Check sheet for the drawn part. Datum: minimum x, y, z corner. Units: mm. A direction names the side the tool comes from. Give positions to 0.01 mm unless a question says otherwise; leave off trailing zeros. Order: outer loops, then holes, each group sorted by start corner. A loop starts at its lowest first (then second) coordinate and runs counter-clockwise, first axis right, second up.
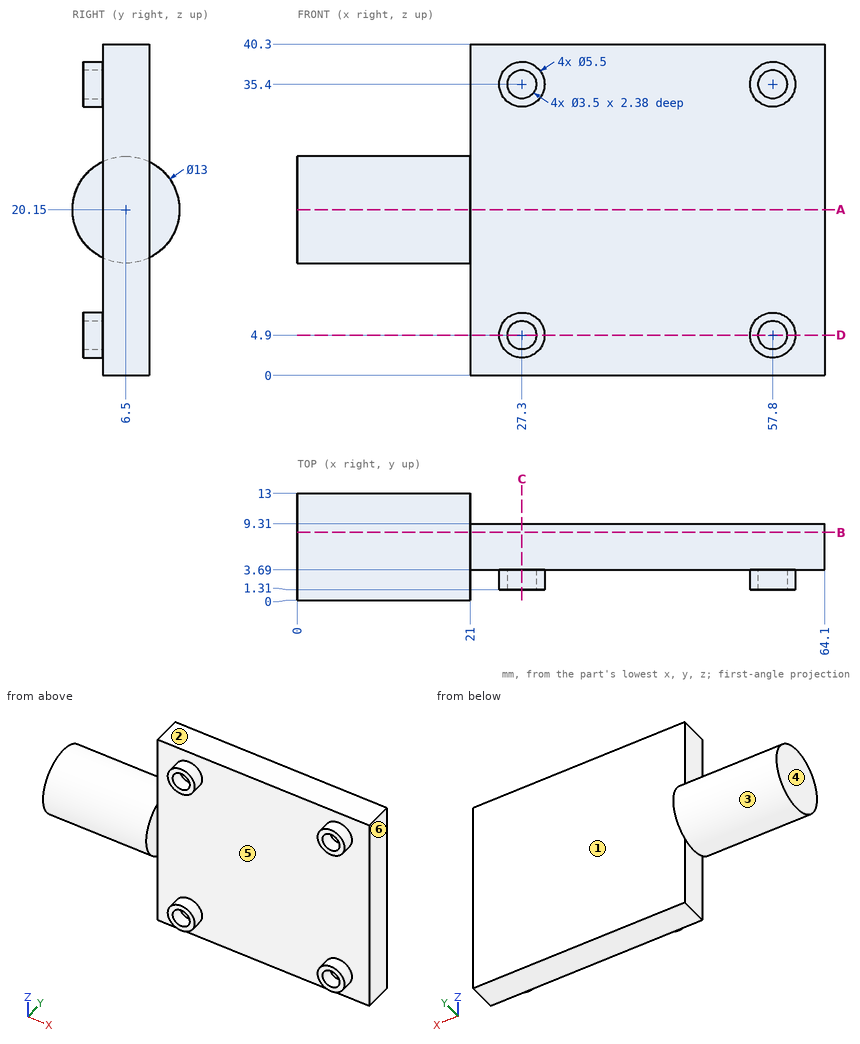
(1) Set-up check for the marked faces 1, 2 and 3: record each of +Z, -Z, +X, -X, +Y, -Y from which the full face is reachable in a straight line by a thin tool's end or side.
Solved:
face 1: +Z, -Z, +X, +Y
face 2: +Z, +X, -X, +Y, -Y
face 3: -X
(2) Section check B-B, the plane y = 8.25. Enter the section's corners in (x, z).
Solved:
outline: (0, 13.89) - (21, 13.89) - (21, 0) - (64.1, 0) - (64.1, 40.3) - (21, 40.3) - (21, 26.41) - (0, 26.41) - close
(3) Go/stop test with flat-tipped pins: pin 1 (2 mm diameter, centred on x = 10, z = 21, fed in from +Y); pin 2 (3 mm diameter, centred on x = 57.5, z = 35, fed in from -Y); pin 3 (5.5 mm diameter, centred on x = 27.3, z = 4.9, fed in from +Y); pin 4 (1.5 mm diameter, centred on y = 8.5, z = 10, fed in from -X). Record where each tip stops, or that it passes through.
Solved:
pin 1: stops at y = 13
pin 2: stops at y = 1.31
pin 3: stops at y = 9.31
pin 4: stops at x = 21
(4) Section check C-C, the plane x = 27.3. Enter the section's corners in (y, z).
Solved:
outline: (1.31, 2.15) - (3.69, 2.15) - (3.69, 0) - (9.31, 0) - (9.31, 40.3) - (3.69, 40.3) - (3.69, 38.15) - (1.31, 38.15) - (1.31, 37.15) - (3.69, 37.15) - (3.69, 33.65) - (1.31, 33.65) - (1.31, 32.65) - (3.69, 32.65) - (3.69, 7.65) - (1.31, 7.65) - (1.31, 6.65) - (3.69, 6.65) - (3.69, 3.15) - (1.31, 3.15) - close
(5) Scan lines: line 1 (Z direction, x = 57.8, y = 2.25); line 2 (X direction, y = 2.4, z = 4.9); line 3 (Y direction, x = 50, z = 25). Record each from-to range of solid material in increasing order.
Solved:
line 1: z = 2.15 to 3.15, 6.65 to 7.65, 32.65 to 33.65, 37.15 to 38.15
line 2: x = 24.55 to 25.55, 29.05 to 30.05, 55.05 to 56.05, 59.55 to 60.55
line 3: y = 3.69 to 9.31
(6) Section check D-D, the plane z = 4.9. Enter the section's corners in (x, y).
Solved:
outline: (21, 3.69) - (24.55, 3.69) - (24.55, 1.31) - (25.55, 1.31) - (25.55, 3.69) - (29.05, 3.69) - (29.05, 1.31) - (30.05, 1.31) - (30.05, 3.69) - (55.05, 3.69) - (55.05, 1.31) - (56.05, 1.31) - (56.05, 3.69) - (59.55, 3.69) - (59.55, 1.31) - (60.55, 1.31) - (60.55, 3.69) - (64.1, 3.69) - (64.1, 9.31) - (21, 9.31) - close
(7) Section check A-A, the plane z = 20.15. Enter the section's corners in (x, y), then the cut area to 3 significant figures.
Solved:
outline: (0, 0) - (21, 0) - (21, 3.69) - (64.1, 3.69) - (64.1, 9.31) - (21, 9.31) - (21, 13) - (0, 13) - close
area: 515 mm2
(8) Release check for a two-part mould opening along X. For the marked faces 4, 5 and 6 record: pulls with the +X half, pulls with the -X half, needs draft (parallel to the pull), parting line crosses it, or undercut.
Solved:
face 4: pulls with the -X half
face 5: undercut
face 6: pulls with the +X half
